from build123d import *

# Parameters (mm, degrees)
F0_W     = 82.55
F0_H     = 12.7
F1_DEPTH = 63.5
F2_DEPTH = 25.4
F3_DEPTH = 7.9375
F5_R     = 6.35


with BuildPart() as f1:
    # F0 (on Front) → F1 (new body, symmetric)
    with BuildSketch(Plane.XZ):
        with Locations((0, -3.175)):
            Rectangle(F0_W, F0_H)
    extrude(amount=F1_DEPTH, both=True)

    # F0 (on Front) → F2 (join, symmetric)
    with BuildSketch(Plane.XZ):
        with Locations((0, -3.175)):
            Rectangle(F0_W, F0_H)
        with BuildLine():
            ThreePointArc((53.577404361, 61.7532924078), (53.0857792806, 61.6992166922), (52.5949692711, 61.6381844286))
            add(Edge.make_bspline(
                [(52.5949692711, 61.6381844286), (52.9244758312, 61.6627898631), (53.2519761831, 61.6860233314), (53.577404361, 61.7078821692)],
                knots=[106.6137732969, 106.6137732969, 106.6137732969, 106.6137732969, 107.6063471029, 107.6063471029, 107.6063471029, 107.6063471029], degree=3))
            Line((53.577404361, 61.7078821692), (53.577404361, 61.7532924078))
        make_face()
        Polygon((22.225, 9.525), (-41.275, 9.525), (-41.275, 3.175), (41.275, 3.175), (41.275, 9.525), align=None)
        with BuildLine():
            ThreePointArc((58.0383306755, 61.9252), (55.8051179778, 61.9105955677), (53.577404361, 61.7532924078))
            Line((53.577404361, 61.7532924078), (53.577404361, 61.7078821692))
            add(Edge.make_bspline(
                [(53.577404361, 61.7078821692), (55.1128174226, 61.8110150488), (56.602102301, 61.8835475984), (58.0383306755, 61.9252)],
                knots=[107.6063471029, 107.6063471029, 107.6063471029, 107.6063471029, 112.2894412218, 112.2894412218, 112.2894412218, 112.2894412218], degree=3))
        make_face()
        with BuildLine():
            Line((22.225, 27.0114993424), (22.225, 9.525))
            Line((22.225, 9.525), (41.275, 9.525))
            Line((41.275, 9.525), (41.275, 27.0114993424))
            ThreePointArc((41.275, 27.0114993424), (44.7256171025, 36.8933177284), (53.577404361, 42.4792782844))
            Line((53.577404361, 42.4792782844), (53.577404361, 61.7078821692))
            add(Edge.make_bspline(
                [(52.5949692711, 61.6381844286), (52.9244758312, 61.6627898631), (53.2519761831, 61.6860233314), (53.577404361, 61.7078821692)],
                knots=[106.6137732969, 106.6137732969, 106.6137732969, 106.6137732969, 107.6063471029, 107.6063471029, 107.6063471029, 107.6063471029], degree=3))
            ThreePointArc((52.5949692711, 61.6381844286), (30.8931906622, 50.0405155696), (22.225, 27.0114993424))
        make_face()
        with BuildLine():
            add(Edge.make_bspline(
                [(53.577404361, 61.7078821692), (55.1128174226, 61.8110150488), (56.602102301, 61.8835475984), (58.0383306755, 61.9252)],
                knots=[107.6063471029, 107.6063471029, 107.6063471029, 107.6063471029, 112.2894412218, 112.2894412218, 112.2894412218, 112.2894412218], degree=3))
            Line((53.577404361, 61.7078821692), (53.577404361, 42.4792782844))
            ThreePointArc((53.577404361, 42.4792782844), (55.6500090256, 42.8154751737), (57.7488542769, 42.8752))
            Line((57.7488542769, 42.8752), (78.977404361, 42.8752))
            Line((78.977404361, 42.8752), (78.977404361, 61.9252))
            Line((78.977404361, 61.9252), (58.0383306755, 61.9252))
        make_face()
    extrude(amount=F2_DEPTH, both=True)

    # F0 (on Front) → F3 (join, symmetric)
    with BuildSketch(Plane.XZ):
        with Locations((0, -3.175)):
            Rectangle(F0_W, F0_H)
        with BuildLine():
            add(Edge.make_bspline(
                [(-41.275, 9.525), (-41.3366305688, 40.5237040654), (17.2021979841, 58.9952794856), (52.5949692711, 61.6381844286)],
                knots=[0, 0, 0, 0, 106.6137732969, 106.6137732969, 106.6137732969, 106.6137732969], degree=3))
            Line((-41.275, 9.525), (22.225, 9.525))
            Line((22.225, 9.525), (22.225, 27.0114993424))
            ThreePointArc((22.225, 27.0114993424), (30.8931906622, 50.0405155696), (52.5949692711, 61.6381844286))
        make_face()
        with BuildLine():
            ThreePointArc((53.577404361, 61.7532924078), (53.0857792806, 61.6992166922), (52.5949692711, 61.6381844286))
            add(Edge.make_bspline(
                [(52.5949692711, 61.6381844286), (52.9244758312, 61.6627898631), (53.2519761831, 61.6860233314), (53.577404361, 61.7078821692)],
                knots=[106.6137732969, 106.6137732969, 106.6137732969, 106.6137732969, 107.6063471029, 107.6063471029, 107.6063471029, 107.6063471029], degree=3))
            Line((53.577404361, 61.7078821692), (53.577404361, 61.7532924078))
        make_face()
        Polygon((22.225, 9.525), (-41.275, 9.525), (-41.275, 3.175), (41.275, 3.175), (41.275, 9.525), align=None)
        with BuildLine():
            ThreePointArc((58.0383306755, 61.9252), (55.8051179778, 61.9105955677), (53.577404361, 61.7532924078))
            Line((53.577404361, 61.7532924078), (53.577404361, 61.7078821692))
            add(Edge.make_bspline(
                [(53.577404361, 61.7078821692), (55.1128174226, 61.8110150488), (56.602102301, 61.8835475984), (58.0383306755, 61.9252)],
                knots=[107.6063471029, 107.6063471029, 107.6063471029, 107.6063471029, 112.2894412218, 112.2894412218, 112.2894412218, 112.2894412218], degree=3))
        make_face()
        with BuildLine():
            Line((22.225, 27.0114993424), (22.225, 9.525))
            Line((22.225, 9.525), (41.275, 9.525))
            Line((41.275, 9.525), (41.275, 27.0114993424))
            ThreePointArc((41.275, 27.0114993424), (44.7256171025, 36.8933177284), (53.577404361, 42.4792782844))
            Line((53.577404361, 42.4792782844), (53.577404361, 61.7078821692))
            add(Edge.make_bspline(
                [(52.5949692711, 61.6381844286), (52.9244758312, 61.6627898631), (53.2519761831, 61.6860233314), (53.577404361, 61.7078821692)],
                knots=[106.6137732969, 106.6137732969, 106.6137732969, 106.6137732969, 107.6063471029, 107.6063471029, 107.6063471029, 107.6063471029], degree=3))
            ThreePointArc((52.5949692711, 61.6381844286), (30.8931906622, 50.0405155696), (22.225, 27.0114993424))
        make_face()
        with BuildLine():
            add(Edge.make_bspline(
                [(53.577404361, 61.7078821692), (55.1128174226, 61.8110150488), (56.602102301, 61.8835475984), (58.0383306755, 61.9252)],
                knots=[107.6063471029, 107.6063471029, 107.6063471029, 107.6063471029, 112.2894412218, 112.2894412218, 112.2894412218, 112.2894412218], degree=3))
            Line((53.577404361, 61.7078821692), (53.577404361, 42.4792782844))
            ThreePointArc((53.577404361, 42.4792782844), (55.6500090256, 42.8154751737), (57.7488542769, 42.8752))
            Line((57.7488542769, 42.8752), (78.977404361, 42.8752))
            Line((78.977404361, 42.8752), (78.977404361, 61.9252))
            Line((78.977404361, 61.9252), (58.0383306755, 61.9252))
        make_face()
    extrude(amount=F3_DEPTH, both=True)

    # F0 (on Front) → F4 (revolve)
    with BuildSketch(Plane.XZ):
        Polygon((104.377404361, 66.675), (78.977404361, 66.675), (78.977404361, 61.9252), (78.977404361, 42.8752), (78.977404361, 38.1), (104.377404361, 38.1), align=None)
    revolve(axis=Axis((78.977404361, 0, 52.3875), (0, 0, 1)))

    # F5
    f5_edges = [f1.edges().sort_by_distance(p)[0] for p in [
        (41.275, -63.5, -3.175),
        (-41.275, -63.5, -3.175),
        (41.275, 63.5, -3.175),
        (-41.275, 63.5, -3.175),
    ]]
    fillet(f5_edges, radius=F5_R)


solid = f1.part
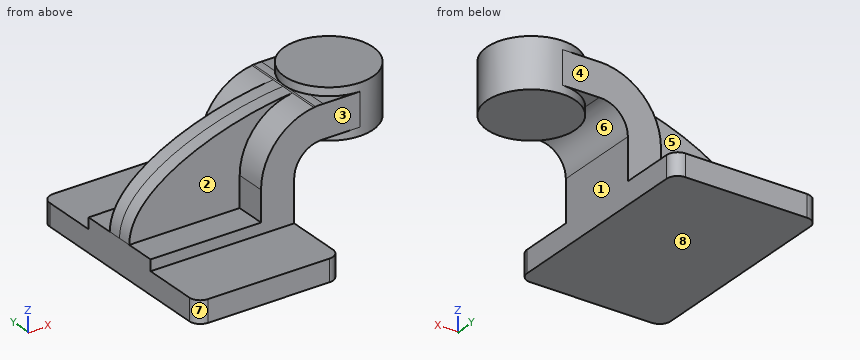
Input: part model. Units: mm. Frame: model coordinates. Face numbers are marked on the shaded views. A direction names the side the tool comes from. Give positions to 0.01 mm unless a question says otherwise; leave off trailing zeros. Order: outer loops, then holes, each group sorted by start corner. A loop starts at its lowest first (then second) coordinate and runs counter-clockwise, first axis right, second up. Notation, with made-up numbers: (-23, -12.75) - (29, -12.75) arc R20 ccw to (29, 20.25) - close; hole circle Ø4 at (49.5, 24). An arc over 180 degrees is marked (long way). Answer as a JSON object with one key per item and string values. Group by question number.
Q1. Line query: probe 1 along Y at (x, z) = (58.5, 59); probe 2 along Z at (x, y) = (9, 36) (3 decimals); probe 3 along Z at (x, y) = (-5, 21.5) (3 decimals). Output: solid intervals per line, ascending.
Q2. Cut plane A-A, the plane z = -0.5. Output: boundary loops of the cut face in (x, y) (3 decimals).
Q3. Mould query, pull axis X, two halves, no side actions, for the marked faces 6, 7 and 8. Classes: pulls with the +X half, pulls with the -X half, needs draft (parallel to the pull), parting line crosses it, or undercut.
Q4. Cut plane B-B, the plane y = -34.5. Output: boundary loops of the cut face in (x, z) (3 decimals).
Q5. Set-up query: the marked faces 1, 2, 3, 4 and 5. Return all of +Z, -Z, +X, -X, +Y, -Y with unobstructed straight access to the full face (end or side cutting, diameter ignored); none if empty.
Q6. First-contact query: pin 1 Ø8 at (x, z) = (86, 34.5) entering from +Y; pin 2 Ø19 at (x, y) = (-15.5, -16.5) entering from +Z; pin 3 Ø5 at (x, y) = (-22, -3.5) entering from +Z; pin 4 Ø8 at (x, y) = (43, -32.5) entering from -Z (3 decimals). Flat tips, straight axial feed; report the tip coordinate or a pass-through.
Results:
{
 "1": {"probe 1": "-25.4 to 25.4", "probe 2": "-9.525 to 3.175", "probe 3": "-9.525 to 9.525"},
 "2": {"outline": "(-41.275, -57.15) arc R6.35 ccw to (-34.925, -63.5) - (34.925, -63.5) arc R6.35 ccw to (41.275, -57.15) - (41.275, 57.15) arc R6.35 ccw to (34.925, 63.5) - (-34.925, 63.5) arc R6.35 ccw to (-41.275, 57.15) - close"},
 "3": {"face 6": "undercut", "face 7": "pulls with the -X half", "face 8": "needs draft"},
 "4": {"outline": "(-41.275, -9.525) - (41.275, -9.525) - (41.275, 3.175) - (-41.275, 3.175) - close"},
 "5": {"face 1": "-Z, +X, +Y, -Y", "face 2": "+Z, -X, -Y", "face 3": "+Z, +X, -X, -Y", "face 4": "+Z, +X, -X, +Y", "face 5": "+Z, -X, +Y"},
 "6": {"pin 1": "y = 24.85", "pin 2": "z = 44.4", "pin 3": "z = 39.85", "pin 4": "z = -9.525"}
}
